Check sheet for the modelled part. Datum: model origin and axes. Units: mm. Coordinates: 2 decimals unless noted, no trailing zeros. Loops run counter-clockwise (first coordinate to the right, second up) from the corner with the lowest first, then second, coordinate; pieces in that order, holes last. Notation, with made-up numbers: (-24, 38.25) -> (-17, 38.25) arc R25 cw to (-17, 69.25) -> close; hole circle Ø10 at (85, -25.75). An arc over 180 degrees is marked (long way). Use CSV: the item, a comma, the result in double quotes. Start each with the question number.
1. Sectioned sample at B-B, the plane x = 6. Record the cut outline in (y, z).
2. Thickness scan on L1, parallel to Y at x = 5.25, z = -109.5; L2, parallel to Y at x = 6, z = -99.5; L3, parallel to Y at x = 6, z = -96. Record the ranges inside material, lowest first.
3. Sectioned sample at D-D, the plane z = -55. Record the cut outline in (x, y), and give its area (3 significant figures).
4. Sectioned sample at C-C, the plane y = 53.5. Record the cut outline in (x, z), and give its area (3 significant figures).
5. Sectioned sample at A-A, the plane z = -29.5. Record the cut outline in (x, y).
6. Release check for a two-part mould opening along Y. For faces 1 (the face through (5, 61, -59)), 2 (the face through (5.1, 22.9, -86.1)), 3 (the face through (10, 34, -34)) record: pulls with the +Y half, pulls with the -Y half, needs draft (parallel to the pull), parting line crosses it, or undercut.
7. Gauge pin test, flat end, axial feed: pin 1 (5 mm diameter, centred on x = 5.5, z = -24.5, fed in from +Y). Record the tip position at first contact, or that the pin passes through.
```python
from build123d import *

# Parameters (mm, degrees)
BOSS_EXTRUDE1_DEPTH = 10
SKETCH4_R           = 2.5
CUT_EXTRUDE3_DEPTH  = 10


with BuildPart() as part:
    # Sketch1 → Boss-Extrude1 (new body)
    with BuildSketch(Plane(origin=(0, 0, 0), x_dir=(0, 0, -1), z_dir=(1, 0, 0))):
        Polygon((0, 0), (0, 120), (120, 0), align=None)
    extrude(amount=BOSS_EXTRUDE1_DEPTH)

    # Sketch4 → Cut-Extrude3 (cut)
    with BuildSketch(Plane(origin=(10, 0, 0), x_dir=(0, 0, -1), z_dir=(1, 0, 0))):
        with Locations((83.720628574, 22.137235802)):
            Circle(SKETCH4_R)
        with Locations((97.862764198, 7.995100178)):
            Circle(SKETCH4_R)
        with Locations((69.578492951, 36.279371426)):
            Circle(SKETCH4_R)
        with Locations((28.991378029, 28.991378029)):
            Circle(SKETCH4_R)
    extrude(amount=-CUT_EXTRUDE3_DEPTH, mode=Mode.SUBTRACT)


solid = part.part
```
Completed:
1,outline,"(0, -120) -> (120, 0) -> (0, 0) -> close; hole circle Ø5 at (8, -97.86); hole circle Ø5 at (22.14, -83.72); hole circle Ø5 at (28.99, -28.99); hole circle Ø5 at (36.28, -69.58)"
2,L1,"0 to 10.5"
2,L2,"0 to 6.11, 9.88 to 20.5"
2,L3,"0 to 6.33, 9.66 to 24"
3,outline,"(0, 0) -> (10, 0) -> (10, 65) -> (0, 65) -> close"
3,area,"650 mm²"
4,outline,"(0, -66.5) -> (10, -66.5) -> (10, 0) -> (0, 0) -> close"
4,area,"665 mm²"
5,outline,"(0, 0) -> (10, 0) -> (10, 26.54) -> (0, 26.54) -> close; (0, 31.44) -> (10, 31.44) -> (10, 90.5) -> (0, 90.5) -> close"
6,face 1,"pulls with the +Y half"
6,face 2,"undercut"
6,face 3,"needs draft"
7,pin 1,"y = 98"
